from build123d import *

# Parameters (mm, degrees)
F0_W     = 304.8
F0_H     = 50.8
F1_DEPTH = 31.75
F2_R     = 5.08
F4_DEPTH = 304.801
F6_DEPTH = 304.8


with BuildPart() as f1:
    # F0 (on Top) → F1 (new body)
    with BuildSketch(Plane.XY):
        Rectangle(F0_W, F0_H)
    extrude(amount=F1_DEPTH)

    # F2
    f2_edges = [f1.edges().sort_by_distance(p)[0] for p in [
        (-152.4, 25.4, 15.875),
        (-152.4, -25.4, 15.875),
        (152.4, 25.4, 15.875),
        (152.4, -25.4, 15.875),
    ]]
    fillet(f2_edges, radius=F2_R)

    # F3 (on face) → F4 (cut, through all)
    with BuildSketch(Plane(origin=(-152.4, 0, 0), x_dir=(0, -1, 0), z_dir=(-1, 0, 0))):
        with BuildLine():
            Line((-25.4, 0), (25.4, 0))
            ThreePointArc((25.4, 0), (0, 25.4), (-25.4, 0))
        make_face()
    extrude(amount=-F4_DEPTH, mode=Mode.SUBTRACT)

    # F5 (on face) → F6 (join, through all)
    with BuildSketch(Plane.YZ.offset(152.4)):
        Polygon((-12.7, 31.75), (0, 31.75), (12.7, 31.75), (19.05, 35.478412), (-19.05, 35.478412), align=None)
    extrude(amount=-F6_DEPTH)


solid = f1.part
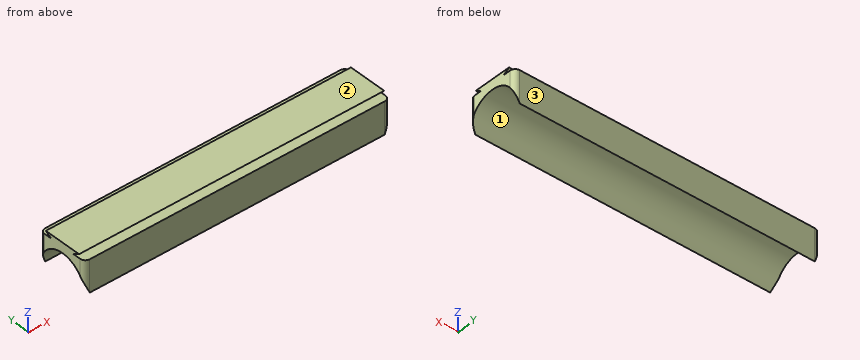
Part model, mm, in its own coordinate system. Face numbers are marked on the shaded views. Give positions to 0.01 mm unless a question says otherwise; leave off trailing zeros. Order: outer loops, then holes, each group sorted by start corner. A loop starts at its lowest first (then second) coordinate and runs counter-clockwise, first axis right, second up. Notation, with made-up numbers: (21.5, 54) - (35.5, 54) arc R31 ccw to (35.5, 89) - close; hole circle Ø11 at (75, 29.5). An arc over 180 degrees is marked (long way). Use a Markdown table: item, result.
1) Saw through at A-A on z = 19.5. List the corners of the cut face in (x, y), plus the area to 3 significant figures.
Checked values:
| item | result |
|---|---|
| outline | (-152.4, -20.32) arc R5.08 ccw to (-147.32, -25.4) - (147.32, -25.4) arc R5.08 ccw to (152.4, -20.32) - (152.4, -16.28) - (-152.4, -16.28) - close; (-152.4, 16.28) - (152.4, 16.28) - (152.4, 20.32) arc R5.08 ccw to (147.32, 25.4) - (-147.32, 25.4) arc R5.08 ccw to (-152.4, 20.32) - close |
| area | 5,540 mm² |
2) Saw through at D-D on y = 0. List the corners of the cut face in (x, z), plus the area to 3 significant figures.
Checked values:
| item | result |
|---|---|
| outline | (-152.4, 25.4) - (152.4, 25.4) - (152.4, 35.48) - (-152.4, 35.48) - close |
| area | 3,070 mm² |
3) Saw through at C-C on y = -15.5. List the corners of the cut face in (x, z), plus the area to 3 significant figures.
Checked values:
| item | result |
|---|---|
| outline | (-152.4, 20.12) - (152.4, 20.12) - (152.4, 31.75) - (-152.4, 31.75) - close; (-152.4, 33.39) - (152.4, 33.39) - (152.4, 35.48) - (-152.4, 35.48) - close |
| area | 4,180 mm² |
4) Two-plate mould, pull along Y, no slides. Class the marked faces 1, 2 and 3: +Y half, -Y half, draft (parallel to the pull), parting line (faces both ways), or undercut.
Checked values:
| item | result |
|---|---|
| face 1 | undercut |
| face 2 | draft |
| face 3 | +Y half |
5) Flat gauge pins, fed straight in: P1, Ø14, axis at x = 5.5, y = -20, coming from the +Z side; P2, Ø1.5, axis at x = 78, y = 17, coming from the -Z side; P3, Ø1.5, axis at x = -26, y = 2, coming from the -Z side; P4, Ø10, axis at x = -62, y = -4.5, coming from the -Z side. Where does each tip first touch, or does it go through?
Checked values:
| item | result |
|---|---|
| P1 | z = 35.48 |
| P2 | z = 18.17 |
| P3 | z = 25.25 |
| P4 | z = 23.56 |
6) Saw through at B-B on x = 16. List the corners of the cut face in (y, z), plus the area to 3 significant figures.
Checked values:
| item | result |
|---|---|
| outline | (-25.4, 0) arc R25.4 cw to (25.4, 0) - (25.4, 31.75) - (12.7, 31.75) - (19.05, 35.48) - (-19.05, 35.48) - (-12.7, 31.75) - (-25.4, 31.75) - close |
| area | 718 mm² |
7) Probe L1, parallel to Z at x = 44, y = -22; L2, parallel to Y at x = 139.5, z = 13.5; L3, parallel to Z at x = -54, y = 15. List the from-to ranges inside material, lowest first. Write a range as from..to.
Checked values:
| item | result |
|---|---|
| L1 | 12.69..31.75 |
| L2 | -25.4..-21.52, 21.52..25.4 |
| L3 | 20.5..31.75, 33.1..35.48 |
